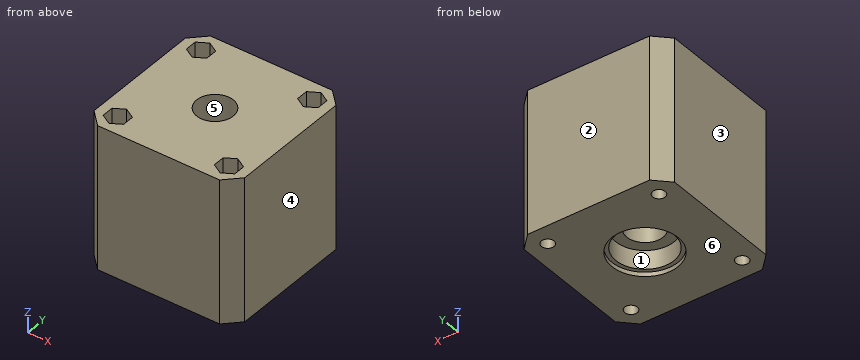
from build123d import *

# Parameters (mm, degrees)
SKETCH_1_W          = 42
SKETCH_1_H          = 42
SKETCH_1_R          = 5.1
SKETCH_1_R_2        = 1.75
EXTRUDE_1_DEPTH     = 40
CHAMFER_1_SIZE      = 4
CUT_EXTRUDE_2_DEPTH = 10
SKETCH_6_R          = 9.2
CUT_EXTRUDE_3_DEPTH = 1.2
SKETCH_7_R          = 8.1
CUT_EXTRUDE_4_DEPTH = 5.2


with BuildPart() as part:
    # 草圖1 → 填料-伸長1 (new body)
    with BuildSketch(Plane.XY):
        Rectangle(SKETCH_1_W, SKETCH_1_H)
        Circle(SKETCH_1_R, mode=Mode.SUBTRACT)
        with Locations((-15.5, 15.5)):
            Circle(SKETCH_1_R_2, mode=Mode.SUBTRACT)
        with Locations(Location((15.5, 15.5, 0), (0, 0, 180))):
            Circle(SKETCH_1_R_2, mode=Mode.SUBTRACT)
        with Locations((15.5, -15.5)):
            Circle(SKETCH_1_R_2, mode=Mode.SUBTRACT)
        with Locations(Location((-15.5, -15.5, 0), (0, 0, 180))):
            Circle(SKETCH_1_R_2, mode=Mode.SUBTRACT)
    extrude(amount=EXTRUDE_1_DEPTH)

    # 導角1
    chamfer_1_edges = [part.edges().sort_by_distance(p)[0] for p in [
        (-21, 21, 20),
        (21, 21, 20),
        (21, -21, 20),
        (-21, -21, 20),
    ]]
    chamfer(chamfer_1_edges, length=CHAMFER_1_SIZE)

    # 草圖5 → 除料-伸長2 (cut)
    with BuildSketch(Plane(origin=(0, 0, 40), x_dir=(-1, 0, 0), z_dir=(0, 0, -1))):
        Polygon((15.5, -12.209103466), (12.65, -13.854551733), (12.65, -17.145448267), (15.5, -18.790896534), (18.35, -17.145448267), (18.35, -13.854551733), align=None)
        Polygon((-15.5, -12.209103466), (-18.35, -13.854551733), (-18.35, -17.145448267), (-15.5, -18.790896534), (-12.65, -17.145448267), (-12.65, -13.854551733), align=None)
        Polygon((-15.5, 12.209103466), (-12.65, 13.854551733), (-12.65, 17.145448267), (-15.5, 18.790896534), (-18.35, 17.145448267), (-18.35, 13.854551733), align=None)
        Polygon((15.5, 12.209103466), (18.35, 13.854551733), (18.35, 17.145448267), (15.5, 18.790896534), (12.65, 17.145448267), (12.65, 13.854551733), align=None)
    extrude(amount=CUT_EXTRUDE_2_DEPTH, mode=Mode.SUBTRACT)

    # 草圖6 → 除料-伸長3 (cut)
    with BuildSketch(Plane(origin=(0, 0, 0), x_dir=(-1, 0, 0), z_dir=(0, 0, -1))):
        Circle(SKETCH_6_R)
    extrude(amount=-CUT_EXTRUDE_3_DEPTH, mode=Mode.SUBTRACT)

    # 草圖7 → 除料-伸長4 (cut)
    with BuildSketch(Plane(origin=(0, 0, 1.2), x_dir=(-1, 0, 0), z_dir=(0, 0, -1))):
        Circle(SKETCH_7_R)
    extrude(amount=-CUT_EXTRUDE_4_DEPTH, mode=Mode.SUBTRACT)


solid = part.part
Could you check a few things on this model? Use its own coordinates, in mm. Face numbers are marked on the shaded views. A direction names the side the tool comes from. Give positions to 0.01 mm unless a question says otherwise; leave off trailing zeros. Write each loop counter-clockwise with the first axis right and the second up, starting at its lowest first coordinate (ties: lowest second). Pieces come first, ordered by that corner, then holes. Notation, with made-up numbers: (8, -19) -> (39, -19) arc R17 ccw to (39, 2) -> close; hole circle Ø8 at (46, 6.25). An arc over 180 degrees is marked (long way). Answer as CSV lines item,"result". Start each with the question number.
(1) If we section it at B-B, the plane z = 31: Give the number of separate pieces and of enclosed holes in the cut face, and give its area (3 significant figures).
(2) Which directions (+Z, -Z, +X, -X, +Y, -Y) give clear straight access to the entire face, cutting with the end or side of a thin tool? Please do the marked faces 1 and 2.
(3) If we section it at C-C, the plane y = 15.5: Write out the boundary of the cut face in (x, z).
(4) Please list where these lines run through material, in increasing order: line 1 (X direction, y = -15.5, z = 15.5); line 2 (Y direction, x = 0, z = 3.05); line 3 (Y direction, x = -15, z = 17).
(5) If we section it at A-A, the plane y = 0: Write out the boundary of the cut face in (x, z).
(6) I'm going to push flat-ended pins straight in: pin 1 Ø2 at (x, y) = (15.5, -15.5) entering from +Z; pin 2 Ø9 at (x, y) = (2.5, -0.5) entering from -Z; pin 3 Ø3 at (x, y) = (-16, 14.5) entering from +Z. Where does each tip first touch, or does it pass through?
(7) If we mould it in two halves opening along X, with no side actions, what happens to the marked faces 3, 4, 5 and 6? For each: +X half, -X half, draft (parallel to the pull), parting line (faces both ways), or undercut.
Answer list:
1,separate pieces,"1"
1,enclosed holes,"5"
1,area,"1,540 mm^2"
2,face 1,"-Z"
2,face 2,"+Z, -Z, +X, -X, +Y"
3,outline,"(-21, 0) -> (-17.25, 0) -> (-17.25, 30) -> (-18.35, 30) -> (-18.35, 40) -> (-21, 40) -> close; (-13.75, 0) -> (13.75, 0) -> (13.75, 30) -> (12.65, 30) -> (12.65, 40) -> (-12.65, 40) -> (-12.65, 30) -> (-13.75, 30) -> close; (17.25, 0) -> (21, 0) -> (21, 40) -> (18.35, 40) -> (18.35, 30) -> (17.25, 30) -> close"
4,line 1,"-21 to -17.25, -13.75 to 13.75, 17.25 to 21"
4,line 2,"-21 to -8.1, 8.1 to 21"
4,line 3,"-21 to -17.18, -13.82 to 13.82, 17.18 to 21"
5,outline,"(-21, 0) -> (-9.2, 0) -> (-9.2, 1.2) -> (-8.1, 1.2) -> (-8.1, 6.4) -> (-5.1, 6.4) -> (-5.1, 40) -> (-21, 40) -> close; (5.1, 6.4) -> (8.1, 6.4) -> (8.1, 1.2) -> (9.2, 1.2) -> (9.2, 0) -> (21, 0) -> (21, 40) -> (5.1, 40) -> close"
6,pin 1,"through"
6,pin 2,"z = 6.4"
6,pin 3,"z = 30"
7,face 3,"-X half"
7,face 4,"+X half"
7,face 5,"undercut"
7,face 6,"draft"
